The model under review builds one solid part; all positions refer to its coordinate system, in mm. A direction names the side the tool comes from. Round coordinates to 2 decimals unless told otherwise and drop trailing zeros. Write each loop counter-clockwise with the first axis right and the second up, starting at its lowest first coordinate (ties: lowest second). Pieces come first, ordered by that corner, then holes.
Item 1: Add section D-D (x = -19.5). Give the boundary of the cut face in (y, z), plus the area to 3 significant figures.
Item 2: Clearance check with flat-ended pins moving along their axes: pin 1 Ø2 at (x, y) = (-3.5, 11) entering from +Z; pin 2 Ø1.5 at (x, y) = (4.5, 14.5) entering from +Z; pin 3 Ø6.5 at (x, y) = (-15.5, 29.5) entering from -Z. State where each tip first meets the part, or that it passes through.
Item 3: Add section A-A (y = 36.5). Give the boundary of the cut face in (x, z) (3 decimals).
Item 4: Add section B-B (z = -11). Give the boundary of the cut face in (x, y).
Item 5: Draft analysis for pull direction X (two halves, no side actions). For faces 1 (the face through (2, 0.573, 3)), 2 (the face through (18.73, 22.49, 17.53)), 3 (the face through (4.636, 40.194, 4.34)), state which applies: +X half, -X half, draft (parallel to the pull), parting line (faces both ways), or undercut.
Item 6: To check wall thickness, follow L1, parallel to Z at x = 2.5, y = 2.5; L2, parallel to Y at x = 4, z = -19; L3, parallel to X at y = 10.5, z = 16. State the ranges of each line that lie inside material, in increasing order.
Item 7: Machinability: for faces 4 (the face through (5, 32.323, 5)), 5 (the face through (3, 45.023, 3)), 6 (the face through (16.41, 40.33, 15.36)), 7 (the face through (-6, 23, 0)), which of the approach directions +Z, -Z, +X, -X, +Y, -Y give a long, thin tool a straight path to every point of the face, cutting with its end or side? Answer none if there is none.
Item 8: Add section C-C (x = 4). Give the boundary of the cut face in (y, z), plus the area to 3 significant figures.
```python
from build123d import *

# Parameters (mm, degrees)
REVOLVE2_ANGLE     = 270
SKETCH5_R          = 3.175
CUT_EXTRUDE1_DEPTH = 46.023434974


with BuildPart() as part:
    # Sketch1 → Revolve2 (revolve)
    with BuildSketch(Plane(origin=(0, 0, 0), x_dir=(0, 0, -1), z_dir=(1, 0, 0))):
        Polygon((22.479, 35.498434974), (22.479, 45.023434974), (25.654, 45.023434974), (25.654, 0.573434974), (22.479, 0.573434974), (22.479, 32.323434974), (6.35, 32.323434974), (6.35, 0.573434974), (3.175, 0.573434974), (3.175, 45.023434974), (6.35, 45.023434974), (6.35, 35.498434974), align=None)
    revolve(axis=Axis((0, 45.023434974, 0), (0, -1, 0)), revolution_arc=REVOLVE2_ANGLE)

    # Sketch5 → Cut-Extrude1 (cut, through all)
    with BuildSketch(Plane(origin=(0, 0, 0), x_dir=(1, 0, 0), z_dir=(0, 1, 0))):
        with Locations((0, 12.7)):
            Circle(SKETCH5_R)
    extrude(amount=CUT_EXTRUDE1_DEPTH, mode=Mode.SUBTRACT)


solid = part.part
```
Numbers:
1. outline: (0.57, 11.18) - (32.32, 11.18) - (32.32, 0) - (35.5, 0) - (35.5, 11.18) - (45.02, 11.18) - (45.02, 16.67) - (0.57, 16.67) - close
1. area: 279 mm2
2. pin 1: stops at z = 25.53
2. pin 2: stops at z = 25.38
2. pin 3: stops at z = 0
3. outline: (-25.654, 0) - (-22.479, 0) arc R22.479 cw (long way) to (0, -22.479) - (0, -25.654) arc R25.654 ccw (long way) to start; (-6.35, 0) - (-3.175, 0) arc R3.175 cw (long way) to (0, -3.175) - (0, -6.35) arc R6.35 ccw (long way) to start
4. outline: (2.68, 32.32) - (19.6, 32.32) - (19.6, 0.57) - (23.18, 0.57) - (23.18, 45.02) - (19.6, 45.02) - (19.6, 35.5) - (2.68, 35.5) - close
5. face 1: draft
5. face 2: parting line
5. face 3: undercut
6. L1: z = -25.53 to -22.34, -5.84 to -1.96, 1.96 to 5.84, 22.34 to 25.53
6. L2: y = 32.32 to 35.5
6. L3: x = -20.05 to -15.79, 15.79 to 20.05
7. face 4: -Y
7. face 5: +Z, -Z, +X, -X, +Y
7. face 6: +Y
7. face 7: -Z, -X, +Y, -Y
8. outline: (0.57, -25.34) - (45.02, -25.34) - (45.02, -22.12) - (35.5, -22.12) - (35.5, -4.93) - (45.02, -4.93) - (45.02, 4.93) - (35.5, 4.93) - (35.5, 22.12) - (45.02, 22.12) - (45.02, 25.34) - (0.57, 25.34) - (0.57, 22.12) - (32.32, 22.12) - (32.32, 4.93) - (0.57, 4.93) - (0.57, -4.93) - (32.32, -4.93) - (32.32, -22.12) - (0.57, -22.12) - close
8. area: 834 mm2
